```python
from build123d import *

# Parameters (mm, degrees)
F1_DEPTH = 4
F2_DEPTH = 60
F3_DEPTH = 60
F4_W     = 20
F4_H     = 60
F5_DEPTH = 4


with BuildPart() as f1:
    # F0 (on Front) → F1 (new body, symmetric)
    with BuildSketch(Plane.XZ):
        with BuildLine():
            Line((0, 0.0707786067), (0, 0))
            Line((0, 0), (0, -60))
            Line((0, -60), (340, -94.9689))
            Line((340, -94.9689), (800, -191.6132215183))
            Line((800, -191.6132215183), (800, 0.5707784817))
            Line((800, 0.5707784817), (0.5003536116, 0.5707784817))
            ThreePointArc((0.5003536116, 0.5707784817), (0.1465716521, 0.4244569958), (0, 0.0707786067))
        make_face()
        with BuildLine():
            Line((0, 60), (0, 0.0707786067))
            ThreePointArc((0, 0.0707786067), (0.1465716521, 0.4244569958), (0.5003536116, 0.5707784817))
            Line((0.5003536116, 0.5707784817), (800, 0.5707784817))
            Line((800, 0.5707784817), (795.5003536116, 192.755164923))
            Line((795.5003536116, 192.755164923), (340, 95.539677511))
            Line((340, 95.539677511), (0, 60))
        make_face()
    extrude(amount=F1_DEPTH, both=True)

    # F0 (on Front) → F2 (join, symmetric)
    with BuildSketch(Plane.XZ):
        with BuildLine():
            Line((0, 0.0707786067), (0, 0))
            Line((0, 0), (0, -60))
            Line((0, -60), (340, -94.9689))
            Line((340, -94.9689), (800, -191.6132215183))
            Line((800, -191.6132215183), (800, 0.5707784817))
            Line((800, 0.5707784817), (0.5003536116, 0.5707784817))
            ThreePointArc((0.5003536116, 0.5707784817), (0.1465716521, 0.4244569958), (0, 0.0707786067))
        make_face()
        with BuildLine():
            Line((0, 60), (0, 0.0707786067))
            ThreePointArc((0, 0.0707786067), (0.1465716521, 0.4244569958), (0.5003536116, 0.5707784817))
            Line((0.5003536116, 0.5707784817), (800, 0.5707784817))
            Line((800, 0.5707784817), (795.5003536116, 192.755164923))
            Line((795.5003536116, 192.755164923), (340, 95.539677511))
            Line((340, 95.539677511), (0, 60))
        make_face()
    extrude(amount=F2_DEPTH, both=True)

    # F3 (add, symmetric): a face of the model
    f3_faces = [f1.faces().sort_by_distance(p)[0] for p in [
        (477.468484718, -60, 0.2503652073),
    ]]
    extrude(f3_faces, amount=F3_DEPTH, both=True)

    # F4 (on Front) → F5 (join, symmetric)
    with BuildSketch(Plane.XZ):
        with Locations((-10, -30)):
            Rectangle(F4_W, F4_H)
        with Locations((-10, 30)):
            Rectangle(F4_W, F4_H)
    extrude(amount=F5_DEPTH, both=True)


solid = f1.part
```
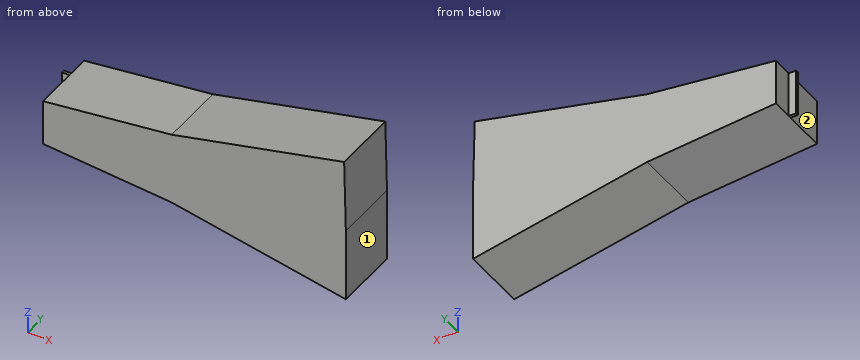
Work out the finished part from the listing and answer in its coordinate system (mm). Face numbers are marked on the shaded views. A direction names the side the tool comes from. Round coordinates to 2 decimals unless told otherwise and drop trailing zeros. Loops run counter-clockwise (first coordinate to the right, second up) from the corner with the lowest first, then second, coordinate; pieces in that order, holes last.
(1) The part is cut by section B-B, the plane z = 163. Give the vertices of the cut face in (x, y), and give its area (3 significant figures).
Computed values:
outline: (656.08, -120) - (796.2, -120) - (796.2, 60) - (656.08, 60) - close
area: 25,200 mm2
(2) For the marked faces 1 and 2, determine the directions among +Z, -Z, +X, -X, +Y, -Y from which every point of the face is accessible in a straight line to the end or side of a thin tool.
Computed values:
face 1: +Z, -Z, +X, +Y, -Y
face 2: +Z, -Z, -X, -Y
(3) The part is cut by section C-C, the plane x = 313.5. Give the vertices of the cut face in (y, z).
Computed values:
outline: (-120, -92.24) - (60, -92.24) - (60, 92.77) - (-120, 92.77) - close
(4) The part is cut by section A-A, the plane y = -90. Give the vertices of the cut face in (x, z).
Computed values:
outline: (0, -60) - (340, -94.97) - (800, -191.61) - (800, 0.57) - (795.5, 192.76) - (340, 95.54) - (0, 60) - close
(5) Each of these flat-tipped pins is pushed along its axis until it touches: P1, Ø2.5, axis at x = -6.5, y = 0.5, coming from the +Z side; P2, Ø16, axis at x = -12.5, z = -14, coming from the +Y side; P3, Ø10, axis at x = -8.5, z = -16, coming from the -Y side. Where does it stop, or does it pass through?
Computed values:
P1: stops at z = 60
P2: stops at y = 4
P3: stops at y = -4
(6) Find the intervals of material crossed by L1, parallel to X at y = -52.5, z = -37; L2, parallel to X at y = -83.5, z = 4; L3, parallel to Z at x = 586.5, y = 10, in increasing order.
Computed values:
L1: x = 0 to 800
L2: x = 0 to 799.92
L3: z = -146.76 to 148.15
